For this review, use the dimensioned drawing (mm, ordinates from the lowest corner) and the shaded views. A direction names the side the tool comes from. Round coordinates to 2 decimals unless told otherwise and drop trailing zeros. Order: outer loops, then holes, each group sorted by start corner. A loop starts at its lowest first (then second) coordinate and runs counter-clockwise, first axis right, second up. Notation, with made-up numbers: (73, 52) - (114, 52) arc R25 ccw to (114, 87) - close; hole circle Ø9 at (88, 15.25). An arc over 180 degrees is marked (long way). Write each question's results on one line, items separated by ' | '. Start each with the question number.
(1) Draft analysis for pull direction Y (two halves, no side actions). For the marked faces 1, 2, 3 and 4, state which applies: pulls with the +Y half, pulls with the -Y half, needs draft (parallel to the pull), parting line crosses it, or undercut.
(2) Take a section at A-A, the plane x = 8. Give the boundary of the cut face in (y, z) (3 decimals).
(3) Insertion check: pin 1 Ø1 at (x, z) = (18, 2) entering from +Y (3 decimals). The pin has a flat end and moves straight along its axis. Give the tip position at first contact, or say it passes through.
(4) For the marked faces 5 and 6, list the 3-axis set-ups (+Z, -Z, +X, -X, +Y, -Y) from which the entire face can be reached by the end or side of a thin tool; tool diameter is ignored.
(5) Take a section at D-D, the plane y = 41.5. Give the boundary of the cut face in (x, z) (3 decimals), plus the area to 3 significant figures.
(6) For L1, parallel to Y at x = 35.5, z = 1.35 (1 decimal); L2, parallel to X at y = 38, z = 2.15 (1 decimal); L3, parallel to X at y = 7, z = 0.6 (1 decimal), list the stretches that pass through material, from the lowest coordinate up. Write a range as from..to.
(7) Take a section at B-B, the plane z = 1.65. Give the boundary of the cut face in (x, y).
(8) Take a section at C-C, the plane y = 23.5. Give the boundary of the cut face in (x, z) (3 decimals).
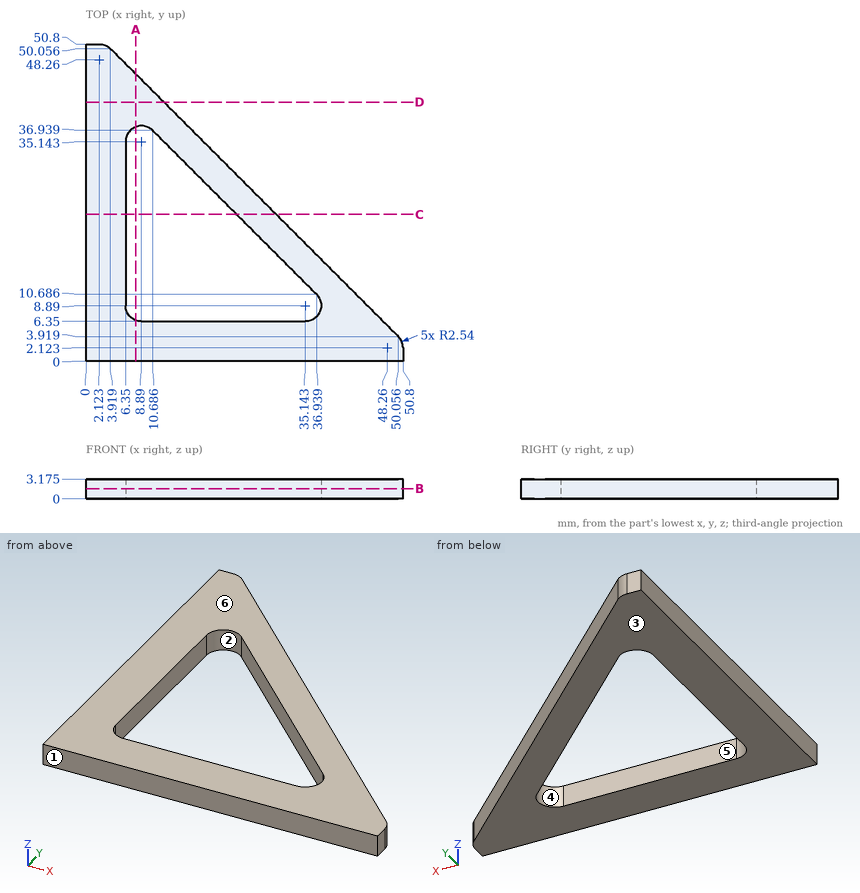
Results below:
1) face 1: pulls with the -Y half | face 2: undercut | face 3: needs draft | face 4: undercut
2) outline: (0, 0) - (6.511, 0) - (6.511, 3.175) - (0, 3.175) - close; (37.522, 0) - (45.975, 0) - (45.975, 3.175) - (37.522, 3.175) - close
3) pin 1: stops at y = 36.475
4) face 5: +Z, -Z | face 6: +Z, +X, -X, +Y, -Y
5) outline: (0, 0) - (12.475, 0) - (12.475, 3.175) - (0, 3.175) - close | area: 39.6 mm^2
6) L1: y = 0..6.4, 12.1..18.5 | L2: x = 0..16 | L3: x = 0..7.2, 36.8..47
7) outline: (0, 0) - (50.8, 0) - (50.8, 2.12) arc R2.54 ccw to (50.06, 3.92) - (3.92, 50.06) arc R2.54 ccw to (2.12, 50.8) - (0, 50.8) - close; hole (6.35, 8.89) arc R2.54 ccw to (8.89, 6.35) - (35.14, 6.35) arc R2.54 ccw to (36.94, 10.69) - (10.69, 36.94) arc R2.54 ccw to (6.35, 35.14) - close
8) outline: (0, 0) - (6.35, 0) - (6.35, 3.175) - (0, 3.175) - close; (24.125, 0) - (30.475, 0) - (30.475, 3.175) - (24.125, 3.175) - close
